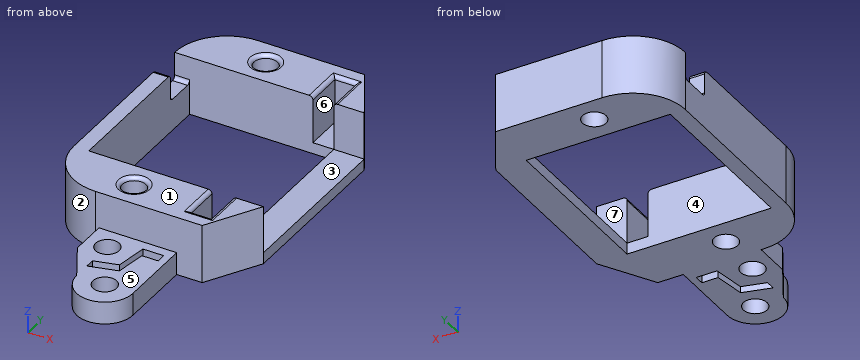
from build123d import *

# Parameters (mm, degrees)
PAD_DEPTH         = 6.35
SKETCH001_W       = 19.26
SKETCH001_H       = 23
PAD001_DEPTH      = 1.5
SKETCH003_R       = 1.58
POCKET_DEPTH      = 92.53341
POCKET_DEPTH_BACK = 97.38341
SKETCH002_W       = 4.4
SKETCH002_H       = 3.6
POCKET001_DEPTH   = 14.106
SKETCH004_R       = 1.58
PAD002_DEPTH      = 3
FILLET_R          = 7
FILLET001_R       = 0.5


with BuildPart() as part:
    # Sketch → Pad (new body)
    with BuildSketch(Plane.XY):
        Polygon((4.355, -11.5), (-12.105, -11.5), (-12.105, 11.5), (4.355, 11.5), (4.355, 16.5), (7.155, 16.5), (7.155, 11.5), (11.215, 11.5), (7.155, 18.5), (-14.105, 18.5), (-14.105, -18.5), (7.155, -18.5), (11.215, -11.5), (7.155, -11.5), (7.155, -16.5), (4.355, -16.5), align=None)
    extrude(amount=PAD_DEPTH)

    # Sketch001 → Pad001 (join)
    with BuildSketch(Plane.XY):
        Polygon((-14.105, 0), (-14.105, 18.5), (7.155, 18.5), (11.215, 11.5), (11.215, -11.5), (7.155, -18.5), (-14.105, -18.5), align=None)
        with Locations((-2.475, 0)):
            Rectangle(SKETCH001_W, SKETCH001_H, mode=Mode.SUBTRACT)
    extrude(amount=-PAD001_DEPTH)

    # Sketch003 → Pocket (cut, two sides)
    with BuildSketch(Plane.XY) as pocket_sk:
        with Locations((-4, 15)):
            Circle(SKETCH003_R)
    pocket = extrude(amount=-POCKET_DEPTH, mode=Mode.SUBTRACT) + extrude(pocket_sk.sketch, amount=POCKET_DEPTH_BACK, mode=Mode.SUBTRACT)

    # Mirrored: Pocket across Sketch003 H_Axis
    add(pocket.mirror(Plane.ZX), mode=Mode.SUBTRACT)

    # Sketch002 → Pocket001 (cut, through all)
    with BuildSketch(Plane.YZ):
        with Locations((9.3, 4.55)):
            Rectangle(SKETCH002_W, SKETCH002_H)
    extrude(amount=-POCKET001_DEPTH, mode=Mode.SUBTRACT)

    # Sketch004 → Pad002 (join)
    with BuildSketch(Plane.XY.offset(-1.5)):
        with BuildLine():
            Line((-6.641136, -18.5), (3.75, -18.5))
            Line((3.75, -18.5), (3.75, -28.5))
            ThreePointArc((-3.75, -28.5), (0, -32.25), (3.75, -28.5))
            Line((-3.75, -28.5), (-6.641136, -23.414276))
            Line((-6.641136, -23.414276), (-6.641136, -18.5))
        make_face()
        with Locations((0, -28.5)):
            Circle(SKETCH004_R, mode=Mode.SUBTRACT)
        with Locations((-3.75, -21.5)):
            Circle(SKETCH004_R, mode=Mode.SUBTRACT)
        Polygon((2.788238, -19.805846), (0, -19.805846), (-0.638352, -24.059963), (-3.75, -24.893727), (-3.75, -26.170431), (0, -25.165621), (0.612686, -21.08255), (2.788238, -21.08255), align=None, mode=Mode.SUBTRACT)
    extrude(amount=PAD002_DEPTH)

    # Fillet
    fillet_edges = [part.edges().sort_by_distance(p)[0] for p in [
        (-14.105, 18.5, 3.175),
        (-14.105, -18.5, 3.175),
    ]]
    fillet(fillet_edges, radius=FILLET_R)

    # Fillet001
    fillet001_edges = [part.edges().sort_by_distance(p)[0] for p in [
        (-5.58, 15, 6.35),
        (-5.58, -15, 6.35),
        (7.155, -14, 6.35),
        (4.355, -14, 6.35),
        (5.755, -16.5, 6.35),
        (4.355, 14, 6.35),
        (5.755, 16.5, 6.35),
        (7.155, 14, 6.35),
        (-13.105, 7.1, 6.35),
        (-13.105, 7.1, 2.75),
        (-13.105, 11.5, 2.75),
    ]]
    fillet(fillet001_edges, radius=FILLET001_R)


solid = part.part
For this review, take the finished solid that the model builds, in its own axes (mm). Face numbers are marked on the shaded views. A direction names the side the tool comes from. Coordinates: 2 decimals unless noted, no trailing zeros. Order: outer loops, then holes, each group sorted by start corner. A loop starts at its lowest first (then second) coordinate and runs counter-clockwise, first axis right, second up. Notation, with made-up numbers: (66.5, 36) - (107.5, 36) arc R20 ccw to (107.5, 69) - close; hole circle Ø5 at (-26, 79.25). An arc over 180 degrees is marked (long way). Answer as CSV lines item,"result". Start each with the question number.
1) Insertion check: P1, Ø1.5, axis at y = 15, z = 4, coming from the +X side; P2, Ø1.5, axis at x = -2, y = -27, coming from the +Z side; P3, Ø0.9, axis at y = -22, z = -0.5, coming from the -X side. Each pin has a flat end and moves straight along its axis. Give the tip position at first contact, or say it passes through.
2) Add section D-D (x = 9). State the section outline as (y, z) points, then the cut area to 3 significant figures.
3) Draft analysis for pull direction Y (two halves, no side actions). For the marked faces 1, 2 and 3, state which applies: +Y half, -Y half, draft (parallel to the pull), parting line (faces both ways), or undercut.
4) Machinability: for the marked faces 4, 5, 6 and 7, which of the approach directions +Z, -Z, +X, -X, +Y, -Y give a long, thin tool a straight path to every point of the face, cutting with its end or side? Answer none if there is none.
5) Add section B-B (x = -4.75). Count the separate pieces of the cut face and the enclosed holes in it, then the cut area to 3 significant figures.
6) Add section C-C (y = -15). State the section outline as (x, z) points (3 decimals).
7) Add section A-A (y = -5). State the section outline as (x, z) points (3 decimals).
8) To check wall thickness, follow line 1 along Y through (x, z) = (-4, 2.75); line 2 along Y through (x, z) = (-4, 0); line 3 along Y through (x, z) = (-2.25, 4.5). State the ranges of each line that lie inside material, in increasing order. Write a range as [from, to].
Result:
1,P1,"x = 9.62"
1,P2,"z = 1.5"
1,P3,"x = -6.64"
2,outline,"(-15.32, -1.5) - (15.32, -1.5) - (15.32, 6.35) - (11.5, 6.35) - (11.5, 0) - (-11.5, 0) - (-11.5, 6.35) - (-15.32, 6.35) - close"
2,area,"94.5 mm^2"
3,face 1,"draft"
3,face 2,"-Y half"
3,face 3,"undercut"
4,face 4,"+Z, -Z"
4,face 5,"+Z, +X, -X, -Y"
4,face 6,"+Z"
4,face 7,"+Z, +X"
5,separate pieces,"5"
5,enclosed holes,"0"
5,area,"83.4 mm^2"
6,outline,"(-13.167, -1.5) - (-5.58, -1.5) - (-5.58, 5.85) arc R0.5 ccw to (-6.08, 6.35) - (-13.167, 6.35) - close; (-2.42, -1.5) - (9.185, -1.5) - (9.185, 6.35) - (7.655, 6.35) arc R0.5 ccw to (7.155, 5.85) - (7.155, 0) - (4.355, 0) - (4.355, 5.85) arc R0.5 ccw to (3.855, 6.35) - (-1.92, 6.35) arc R0.5 ccw to (-2.42, 5.85) - close"
7,outline,"(-14.105, -1.5) - (-12.105, -1.5) - (-12.105, 6.35) - (-14.105, 6.35) - close; (7.155, -1.5) - (11.215, -1.5) - (11.215, 0) - (7.155, 0) - close"
8,line 1,"[-18.5, -16.58], [-13.42, -11.5], [11.5, 13.42], [16.58, 18.5]"
8,line 2,"[-28.06, -23.06], [-19.94, -16.58], [-13.42, -11.5], [11.5, 13.42], [16.58, 18.5]"
8,line 3,"[-18.5, -11.5], [11.5, 18.5]"
